Read the model definition and answer for the solid it produces. Units are mm, in the model's axes. A direction names the side the tool comes from. Give positions to 0.01 mm unless a question says otherwise; leave off trailing zeros. Order: outer loops, then holes, each group sorted by start corner. A loop starts at its lowest first (then second) coordinate and runs counter-clockwise, first axis right, second up. Notation, with made-up numbers: M 5.25,85.25 L 28.25,85.25 A17 cw 28.25,114.25 Z; hole C -31.75,12 d3. An arc over 180 degrees is marked long. One line per item, written item: value.
from build123d import *

# Parameters (mm, degrees)
CROQUIS1_W              = 350
CROQUIS1_H              = 90
SALIENTE_EXTRUIR1_DEPTH = 70
CROQUIS2_W              = 320
CROQUIS2_H              = 70
CORTAR_EXTRUIR1_DEPTH   = 194.778223751
CROQUIS3_R              = 11.125
CORTAR_EXTRUIR2_DEPTH   = 360.756862339
CROQUIS8_R              = 11.075
CORTAR_EXTRUIR3_DEPTH   = 209.865985742
CROQUIS9_R              = 11.075
CORTAR_EXTRUIR5_DEPTH   = 209.865985742


with BuildPart() as part:
    # Croquis1 → Saliente-Extruir1 (new body)
    with BuildSketch(Plane(origin=(0, 0, 0), x_dir=(1, 0, 0), z_dir=(0, 1, 0))):
        Rectangle(CROQUIS1_W, CROQUIS1_H)
    extrude(amount=SALIENTE_EXTRUIR1_DEPTH)

    # Croquis2 → Cortar-Extruir1 (cut, through all)
    with BuildSketch(Plane(origin=(0, 70, 0), x_dir=(1, 0, 0), z_dir=(0, 1, 0))):
        with Locations((0, -10)):
            Rectangle(CROQUIS2_W, CROQUIS2_H)
    extrude(amount=-CORTAR_EXTRUIR1_DEPTH, mode=Mode.SUBTRACT)

    # Croquis3 → Cortar-Extruir2 (cut, through all)
    with BuildSketch(Plane.ZY.offset(175)):
        with Locations((25, 48)):
            Circle(CROQUIS3_R)
    extrude(amount=-CORTAR_EXTRUIR2_DEPTH, mode=Mode.SUBTRACT)

    # Croquis8 → Cortar-Extruir3 (cut, through all)
    with BuildSketch(Plane(origin=(0, 0, -45), x_dir=(-1, 0, 0), z_dir=(0, 0, -1))):
        with Locations((-143.5, 21.5)):
            Circle(CROQUIS8_R)
    cortar_extruir3 = extrude(amount=-CORTAR_EXTRUIR3_DEPTH, mode=Mode.SUBTRACT)

    # Simetría1: Cortar-Extruir3 across plane
    add(cortar_extruir3.mirror(Plane(origin=(0, 0, 0), x_dir=(0, 0, 1), z_dir=(1, 0, 0))), mode=Mode.SUBTRACT)

    # Croquis9 → Cortar-Extruir5 (cut, through all)
    with BuildSketch(Plane(origin=(0, 0, -45), x_dir=(-1, 0, 0), z_dir=(0, 0, -1))):
        Polygon((-25, 35), (-25, 17.5), (25, 17.5), (25, 0), (175, 0), (175, 70), (-25, 70), (-25, 52.5), (25, 52.5), (25, 35), align=None)
        with Locations((143.5, 21.5)):
            Circle(CROQUIS9_R, mode=Mode.SUBTRACT)
    extrude(amount=-CORTAR_EXTRUIR5_DEPTH, mode=Mode.SUBTRACT)


solid = part.part
1) Which of the six approach directions +Z, -Z, +X, -X, +Y, -Y give full straight-line access (tool end or side, diameter ignored) to faces 1 (the face through (160, 35, 10)), 2 (the face through (-25, 44, -35)), 3 (the face through (0, 52.5, -35)), 4 (the face through (0, 17.5, -35))?
Reported:
face 1: +Z, -X, +Y, -Y
face 2: +Z, -Z, -X, +Y, -Y
face 3: +Z, -Z, -X, +Y
face 4: +Z, -Z, -X
2) Find section C-C, the plane x = 143.5. Write down the section's boundary in (y, z) (3 decimals).
Reported:
outline: M 0,-45 L 10.425,-45 L 10.425,-25 L 0,-25 Z; M 32.575,-45 L 70,-45 L 70,-25 L 32.575,-25 Z
3) Find section D-D, the plane z = -35. Write down the section's boundary in (x, y) (3 decimals), plus the area to 3 significant figures.
Reported:
outline: M -25,0 L 175,0 L 175,70 L 25,70 L 25,52.5 L -25,52.5 L -25,35 L 25,35 L 25,17.5 L -25,17.5 Z; hole C 143.5,21.5 d22.15
area: 11,900 mm^2
4) Find section A-A, the plane y = 21.5. Write down the section's boundary in (x, z) (3 decimals).
Reported:
outline: M 25,-45 L 132.425,-45 L 132.425,-25 L 25,-25 Z; M 154.575,-45 L 175,-45 L 175,45 L 160,45 L 160,-25 L 154.575,-25 Z
5) Each of these flat-tipped pins is pushed along its axis until it touches: pin 1 Ø13.5 at (y, z) = (48, 25) entering from -X; pin 2 Ø6 at (x, z) = (1.5, -32) entering from +Y; pin 3 Ø5 at (x, y) = (132, 59.5) entering from +Z; pin 4 Ø14 at (y, z) = (62.5, -35.5) entering from -X. Where does it stop, or does it pass through?
Reported:
pin 1: passes through
pin 2: stops at y = 52.5
pin 3: stops at z = -25
pin 4: stops at x = 25
6) Determine the mould class of faces 5 (the face through (25, 26, -35)), 6 (the face through (167, 35, 45)), 7 (the face through (167.4, 59.03, 23.55)) for opening direction Z: +Z half, -Z half, draft (parallel to the pull), parting line (faces both ways), or undercut.
Reported:
face 5: draft
face 6: +Z half
face 7: undercut
7) Find section B-B, the plane z = 25. Write down the section's boundary in (x, y) (3 decimals), plus the area to 3 significant figures.
Reported:
outline: M 160,0 L 175,0 L 175,36.875 L 160,36.875 Z; M 160,59.125 L 175,59.125 L 175,70 L 160,70 Z
area: 716 mm^2
8) Consider probe 1 along X at (y, z) = (21, -36); probe 2 along Y at (x, z) = (143.5, -31) (3 decimals); probe 3 along Y at (x, z) = (171, 25) (3 decimals). Determine where each line is inside the solid, lowest interval first.
Reported:
probe 1: x = 25 to 132.44, 154.56 to 175
probe 2: y = 0 to 10.425, 32.575 to 70
probe 3: y = 0 to 36.875, 59.125 to 70
